Model file for the job. Use its own axes, mm. A direction names the side the tool comes from. Round coordinates to 2 decimals unless told otherwise and drop trailing zeros. Write each loop counter-clockwise with the first axis right and the second up, starting at its lowest first coordinate (ties: lowest second). Pieces come first, ordered by that corner, then holes.
```python
from build123d import *

# Parameters (mm, degrees)
CROQUIS1_W                          = 93
CROQUIS1_H                          = 70
SALIENTE_EXTRUIR1_DEPTH             = 1.5
CROQUIS2_W                          = 78
CROQUIS2_H                          = 51
SALIENTE_EXTRUIR2_DEPTH             = 8.6
DI_METRO_DE_TALADRO_3_1_3_1_1_D     = 3.1
DI_METRO_DE_TALADRO_3_1_3_1_1_DEPTH = 10.1
REDONDEO1_R                         = 1
CROQUIS5_W                          = 72
CROQUIS5_H                          = 40
CORTAR_EXTRUIR1_DEPTH               = 1


with BuildPart() as part:
    # Croquis1 → Saliente-Extruir1 (new body)
    with BuildSketch(Plane.XY.offset(6)):
        with Locations((0, 8.5)):
            Rectangle(CROQUIS1_W, CROQUIS1_H)
    extrude(amount=-SALIENTE_EXTRUIR1_DEPTH)

    # Croquis2 → Saliente-Extruir2 (add)
    with BuildSketch(Plane.XY.offset(6)):
        with Locations((-0.2, 8.5)):
            Rectangle(CROQUIS2_W, CROQUIS2_H)
    extrude(amount=SALIENTE_EXTRUIR2_DEPTH)

    # Diámetro de taladro Ø3.1 (3.1)1
    with Locations(Plane(origin=(0, 0, 4.5), x_dir=(-1, 0, 0), z_dir=(0, 0, -1))):
        with Locations((43.95, -23.95), (-43.95, -23.95), (43.95, 40.95), (-43.95, 40.95)):
            Hole(DI_METRO_DE_TALADRO_3_1_3_1_1_D / 2, depth=DI_METRO_DE_TALADRO_3_1_3_1_1_DEPTH)

    # Redondeo1
    redondeo1_edges = [part.edges().sort_by_distance(p)[0] for p in [
        (-0.2, -17, 14.6),
        (38.8, 8.5, 14.6),
        (-0.2, 34, 14.6),
        (-39.2, 8.5, 14.6),
    ]]
    fillet(redondeo1_edges, radius=REDONDEO1_R)

    # Croquis5 → Cortar-Extruir1 (cut)
    with BuildSketch(Plane.XY.offset(14.6)):
        with Locations((-0.2, 8.5)):
            Rectangle(CROQUIS5_W, CROQUIS5_H)
    extrude(amount=-CORTAR_EXTRUIR1_DEPTH, mode=Mode.SUBTRACT)


solid = part.part
```
1) Which spindle directions (+Z, -Z, +X, -X, +Y, -Y) get a long thin tool onto all of the face, cutting with end or side? Do faces 1 (the face through (-39.2, 8, 10)), 2 (the face through (38.8, 8, 10)), 3 (the face through (-1, -17, 10)), 4 (the face through (42.4, -23.9, 5.3)), 5 (the face through (-1, 9, 13.6)). Say none if no direction does.
2) Cut at D-D on y = 21.5. List the corners of the cut face in (x, z).
3) Cut at A-A on x = -43.95. List the corners of the cut face in (y, z), and give its area (3 significant figures).
4) Wall check: probe 1 along Y at (x, z) = (-43.95, 5.1); probe 2 along Z at (x, y) = (9.5, 14); probe 3 along X at (y, z) = (24, 14.25). Give the ranges that are in metal, low to high.
5) Pull direction Y, two halves, no side cores. Call faces 6 (the face through (-1, 34, 10)), 7 (the face through (-1, -22, 6)), 8 (the face through (-45.5, -23.9, 5.3)): released by +Y, released by -Y, zero draft, split by the parting line, or undercut.
6) Cut at C-C on x = 27. List the corners of the cut face in (y, z), and give its area (3 significant figures).
7) Cut at B-B on y = 40.95. List the corners of the cut face in (x, z).
8) Flat gauge pins, fed straight in: pin 1 Ø0.8 at (y, z) = (18.5, 14) entering from -X; pin 2 Ø6 at (y, z) = (10, 11.5) entering from +X; pin 3 Ø1.1 at (x, z) = (5, 14) entering from +Y. Where does each tip first touch, or does it go through?
Result sheet:
1. face 1: +Z, -X, +Y, -Y
1. face 2: +Z, +X, +Y, -Y
1. face 3: +Z, +X, -X, -Y
1. face 4: +Z, -Z
1. face 5: +Z
2. outline: (-46.5, 4.5) - (46.5, 4.5) - (46.5, 6) - (38.8, 6) - (38.8, 13.6) arc R1 ccw to (37.8, 14.6) - (35.8, 14.6) - (35.8, 13.6) - (-36.2, 13.6) - (-36.2, 14.6) - (-38.2, 14.6) arc R1 ccw to (-39.2, 13.6) - (-39.2, 6) - (-46.5, 6) - close
3. outline: (-26.5, 4.5) - (-25.5, 4.5) - (-25.5, 6) - (-26.5, 6) - close; (-22.4, 4.5) - (39.4, 4.5) - (39.4, 6) - (-22.4, 6) - close; (42.5, 4.5) - (43.5, 4.5) - (43.5, 6) - (42.5, 6) - close
3. area: 95.7 mm2
4. probe 1: y = -26.5 to -25.5, -22.4 to 39.4, 42.5 to 43.5
4. probe 2: z = 4.5 to 13.6
4. probe 3: x = -38.96 to -36.2, 35.8 to 38.56
5. face 6: released by +Y
5. face 7: zero draft
5. face 8: undercut
6. outline: (-26.5, 4.5) - (43.5, 4.5) - (43.5, 6) - (34, 6) - (34, 13.6) arc R1 ccw to (33, 14.6) - (28.5, 14.6) - (28.5, 13.6) - (-11.5, 13.6) - (-11.5, 14.6) - (-16, 14.6) arc R1 ccw to (-17, 13.6) - (-17, 6) - (-26.5, 6) - close
6. area: 503 mm2
7. outline: (-46.5, 4.5) - (-45.5, 4.5) - (-45.5, 6) - (-46.5, 6) - close; (-42.4, 4.5) - (42.4, 4.5) - (42.4, 6) - (-42.4, 6) - close; (45.5, 4.5) - (46.5, 4.5) - (46.5, 6) - (45.5, 6) - close
8. pin 1: stops at x = -39.2
8. pin 2: stops at x = 38.8
8. pin 3: stops at y = 34
